from build123d import *

# Parameters (mm, degrees)
F0_W     = 100
F0_H     = 50
F1_DEPTH = 7.5
F2_R     = 5
F2_W     = 10
F2_H     = 10
F3_DEPTH = 10
F4_R     = 5.5
F5_DEPTH = 1


# Not quite as in the source:
# - a feature names something its author has since deleted; it is built from what else it names


with BuildPart() as f1:
    # F0 (on Front) → F1 (new body, symmetric)
    with BuildSketch(Plane.XZ):
        Rectangle(F0_W, F0_H)
    extrude(amount=F1_DEPTH, both=True)

    # F2 (on face) → F3 (cut)
    with BuildSketch(Plane.XZ.offset(7.5)):
        with Locations((-40, 0)):
            Circle(F2_R)
        with Locations((40, 0)):
            Rectangle(F2_W, F2_H)
    extrude(amount=-F3_DEPTH, mode=Mode.SUBTRACT)

    # F4 (on face) → F5 (cut)
    with BuildSketch(Plane.XZ.offset(-2.5)):
        with Locations((-40, 0)):
            Circle(F4_R)
    extrude(amount=F5_DEPTH, mode=Mode.SUBTRACT)


solid = f1.part
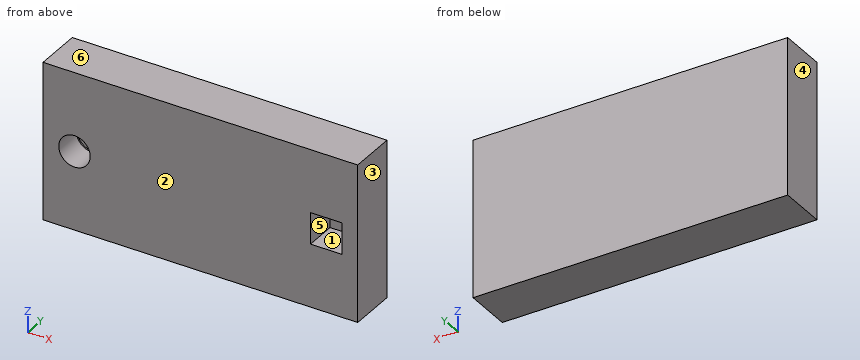
Verification items for the finished model (mm, model axes). Face numbers are marked on the shaded views. A direction names the side the tool comes from. Coordinates: 2 decimals unless noted, no trailing zeros. Order: outer loops, then holes, each group sorted by start corner. A loop starts at its lowest first (then second) coordinate and runs counter-clockwise, first axis right, second up. Notation, with made-up numbers: M 35,-18 L 60,-18 A20 ccw 60,-4 Z; hole C -40,45 d10. An arc over 180 degrees is marked long. One line per item, written item: value. Start each with the question number.
Item 1: Gauge pin test, flat ends, axial feed: pin 1 (5.5 mm diameter, centred on x = -38, z = 0, fed in from -Y); pin 2 (11 mm diameter, centred on x = 39, z = -2, fed in from -Y). Record the tip position at first contact, or that the pin passes through.
Item 2: Sectioned sample at C-C (x = -40). Enter the section's corners in (y, z).
Item 3: Mould release check, pull along X, two halves, no side actions. Record for the marked faces 3, 4, 5 and 6: released by +X, released by -X, zero draft, split by the parting line, or undercut.
Item 4: Scan lines: probe 1 along X at (y, z) = (-3, 2); probe 2 along Z at (x, y) = (-40, -2.75); probe 3 along Z at (x, y) = (-40, 1.95). Record each from-to range of solid material in increasing order.
Item 5: Sectioned sample at B-B (z = 0). Enter the section's corners in (x, y), then the cut area to 3 significant figures.
Item 6: Access from +Z, -Z, +X, -X, +Y, -Y to the whole of each face (thin tool, end or side, straight path). Record for the marked faces 1 and 2.
Item 7: Sectioned sample at A-A (y = -1.5). Enter the section's corners in (x, z).
Conclusion:
1. pin 1: stops at y = 2.5
1. pin 2: stops at y = -7.5
2. outline: M -7.5,-25 L 7.5,-25 L 7.5,25 L -7.5,25 L -7.5,5 L 1.5,5 L 1.5,5.5 L 2.5,5.5 L 2.5,-5.5 L 1.5,-5.5 L 1.5,-5 L -7.5,-5 Z
3. face 3: released by +X
3. face 4: released by -X
3. face 5: undercut
3. face 6: zero draft
4. probe 1: x = -50 to -44.58, -35.42 to 35, 45 to 50
4. probe 2: z = -25 to -5, 5 to 25
4. probe 3: z = -25 to -5.5, 5.5 to 25
5. outline: M -50,-7.5 L -45,-7.5 L -45,1.5 L -45.5,1.5 L -45.5,2.5 L -34.5,2.5 L -34.5,1.5 L -35,1.5 L -35,-7.5 L 35,-7.5 L 35,2.5 L 45,2.5 L 45,-7.5 L 50,-7.5 L 50,7.5 L -50,7.5 Z
5. area: 1,300 mm^2
6. face 1: -Y
6. face 2: +Z, -Z, +X, -X, -Y
7. outline: M -50,-25 L 50,-25 L 50,25 L -50,25 Z; hole C -40,0 d10; hole M 35,-5 L 45,-5 L 45,5 L 35,5 Z
